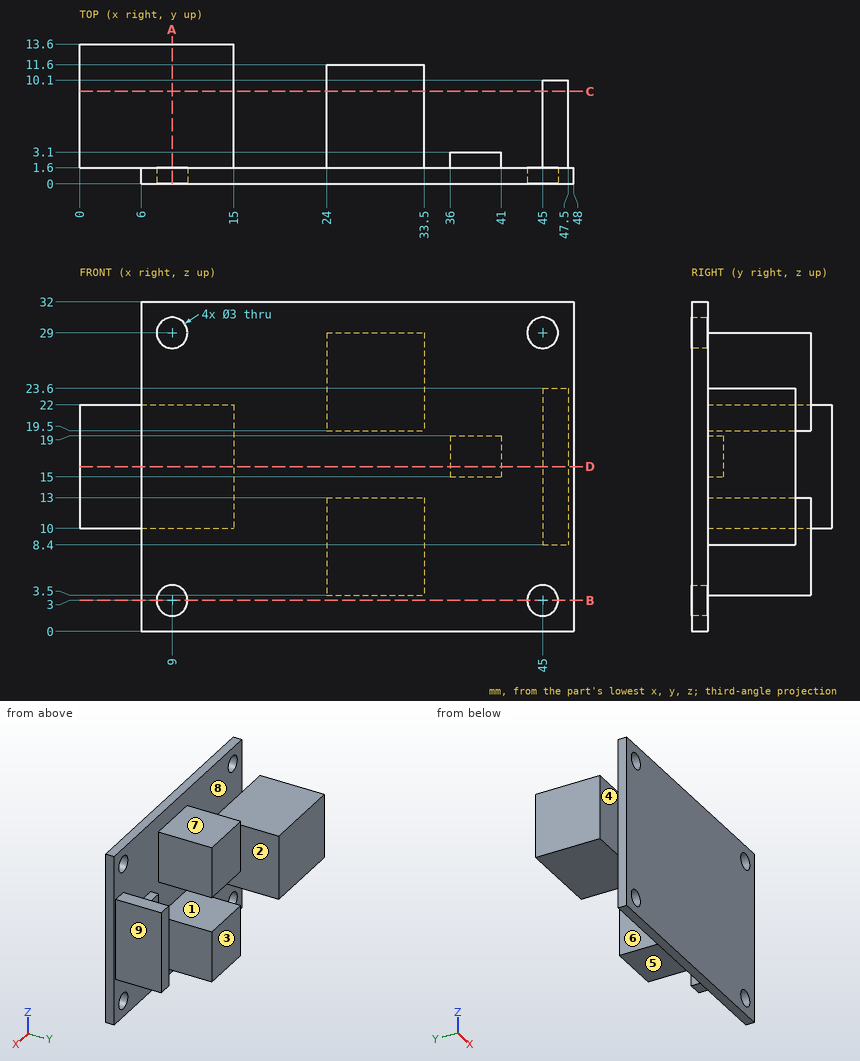
The figure shows three views and two pictorial views of one solid part (mm, origin at its lowest corner). Answer the questions. A direction names the side the tool comes from. Coordinates: 2 decimals unless noted, no trailing zeros. Write each loop counter-clockwise with the first axis right and the second up, starting at its lowest first coordinate (ties: lowest second). Pieces come first, ordered by that corner, then holes.
1. Flat-ended cylindrical pins translate along their axes: pin 1 (1.2 mm diameter, centred on x = 46, z = 15, fed in from +Y); pin 2 (3 mm diameter, centred on x = 2, z = 16.5, fed in from -Y); pin 3 (0.8 mm diameter, centred on y = 1, z = 10, fed in from -X). Find the tip coordinate at first contact, or state that the pin passes through.
Results list:
pin 1: stops at y = 10.1
pin 2: stops at y = 1.6
pin 3: stops at x = 6
2. The part is cut by section D-D, the plane z = 16. Write down the section's boundary in (x, y).
Results list:
outline: (0, 1.6) - (6, 1.6) - (6, 0) - (48, 0) - (48, 1.6) - (47.5, 1.6) - (47.5, 10.1) - (45, 10.1) - (45, 1.6) - (41, 1.6) - (41, 3.1) - (36, 3.1) - (36, 1.6) - (15, 1.6) - (15, 13.6) - (0, 13.6) - close
3. For the marked faces 1, 2, 3, 4 and 5, determine the directions among +Z, -Z, +X, -X, +Y, -Y from which every point of the face is accessible in a straight line to the end or side of a thin tool.
Results list:
face 1: +Y
face 2: +Z, -Z, +Y
face 3: +Z, -Z, +X, +Y
face 4: +Z, -Z, -X, -Y
face 5: -Z, +X, -X, +Y
4. The part is cut by section B-B, the plane z = 3. Write down the section's boundary in (x, y), and give its area (3 significant figures).
Results list:
outline: (6, 0) - (7.5, 0) - (7.5, 1.6) - (6, 1.6) - close; (10.5, 0) - (43.5, 0) - (43.5, 1.6) - (10.5, 1.6) - close; (46.5, 0) - (48, 0) - (48, 1.6) - (46.5, 1.6) - close
area: 57.6 mm2
5. Consider line 1 along X through (y, z) = (0.65, 3); line 2 along Z through (x, y) = (45, 0.7); line 3 along X through (y, z) = (0.5, 2). Determine where each line is inside the solid, lowest interval first.
Results list:
line 1: x = 6 to 7.5, 10.5 to 43.5, 46.5 to 48
line 2: z = 0 to 1.5, 4.5 to 27.5, 30.5 to 32
line 3: x = 6 to 7.88, 10.12 to 43.88, 46.12 to 48
6. For a pull along X with two mould halves and no side action, classify the marked faces 6, 7, 8 and 9 as +X half, -X half, draft (parallel to the pull), parting line (faces both ways), or undercut.
Results list:
face 6: undercut
face 7: draft
face 8: undercut
face 9: +X half
7. The part is cut by section C-C, the plane y = 9. Write down the section's boundary in (x, z), and give its area (4 significant figures).
Results list:
outline: (0, 10) - (15, 10) - (15, 22) - (0, 22) - close; (24, 3.5) - (33.5, 3.5) - (33.5, 13) - (24, 13) - close; (24, 19.5) - (33.5, 19.5) - (33.5, 29) - (24, 29) - close; (45, 8.4) - (47.5, 8.4) - (47.5, 23.6) - (45, 23.6) - close
area: 398.5 mm2
8. The part is cut by section A-A, the plane x = 9. Write down the section's boundary in (y, z).
Results list:
outline: (0, 0) - (1.6, 0) - (1.6, 1.5) - (0, 1.5) - close; (0, 4.5) - (1.6, 4.5) - (1.6, 10) - (13.6, 10) - (13.6, 22) - (1.6, 22) - (1.6, 27.5) - (0, 27.5) - close; (0, 30.5) - (1.6, 30.5) - (1.6, 32) - (0, 32) - close
